Print and shaded views of the part. All mm, measured from the part's lowest x, y and z. A direction names the side the tool comes from. Coordinates: 2 decimals unless noted, no trailing zeros. Order: outer loops, then holes, each group sorted by start corner. A loop starts at its lowest first (then second) coordinate and runs counter-clockwise, first axis right, second up. Notation, with made-up numbers: (50.25, -31) -> (99.25, -31) arc R18 ccw to (99.25, -26) -> close; hole circle Ø4 at (44.5, -9.5). An arc over 180 degrees is marked (long way). Return JSON: item names as keys, results as strings. Group by question number.
1) Probe line 1 (X direction, y = 0.35, z = 4.75); line 2 (Z direction, x = 13, y = 0.8); line 3 (X direction, y = 2.9, z = 1.5). List the from-to ranges inside material, lowest first.
2) Cut at C-C (z = 1.5). Write the cut outline in (x, y), and give its area (3 significant figures).
3) Which spindle directions (+Z, -Z, +X, -X, +Y, -Y) get a long thin tool onto all of the face, cutting with end or side? Do the marked faces 4 and 5. Say none if no direction does.
4) Flat gauge pins, fed straight in: pin 1 (1 mm diameter, centred on y = 2, z = 5.5, fed in from +X); pin 2 (5 mm diameter, centred on x = 9.5, z = 6, fed in from +Y). Where does each tip first touch, or does it go through?
5) Cut at D-D (y = 0.4). Write the cut outline in (x, z), and give its area (3 significant figures).
6) Pull direction X, two halves, no side cores. Call the marked faces 1, 2 and 3: +X half, -X half, draft (parallel to the pull), parting line (faces both ways), or undercut.
7) Cut at B-B (x = 8). Write the cut outline in (y, z), and give its area (3 significant figures).
8) Cut at A-A (z = 4.75). Write the cut outline in (x, y), and give its area (3 significant figures).
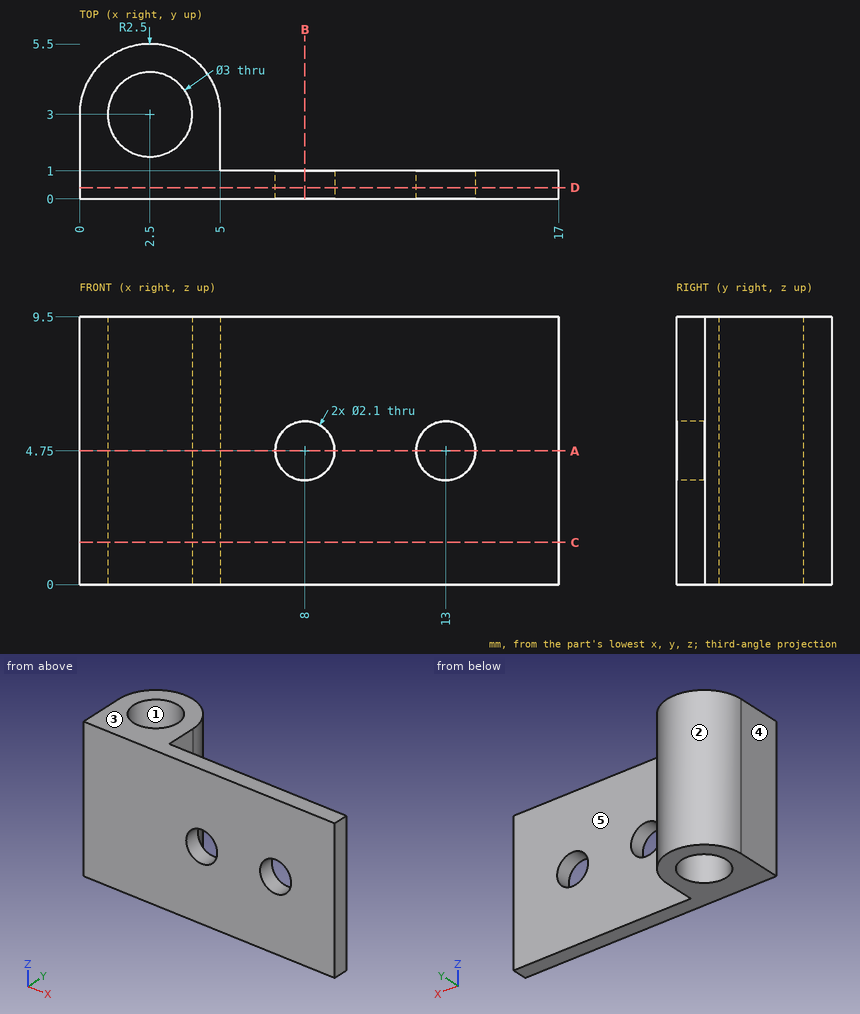
Answers below:
{
 "1": {"line 1": "x = 0 to 6.95, 9.05 to 11.95, 14.05 to 17", "line 2": "z = 0 to 3.7, 5.8 to 9.5", "line 3": "x = 0 to 1, 4 to 5"},
 "2": {"outline": "(0, 0) -> (17, 0) -> (17, 1) -> (5, 1) -> (5, 3) arc R2.5 ccw to (0, 3) -> close; hole circle Ø3 at (2.5, 3)", "area": "29.7 mm^2"},
 "3": {"face 4": "+Z, -Z, -X, +Y, -Y", "face 5": "+Z, -Z, +X, +Y"},
 "4": {"pin 1": "stops at x = 5", "pin 2": "stops at y = 1"},
 "5": {"outline": "(0, 0) -> (17, 0) -> (17, 9.5) -> (0, 9.5) -> close; hole circle Ø2.1 at (8, 4.75); hole circle Ø2.1 at (13, 4.75)", "area": "155 mm^2"},
 "6": {"face 1": "undercut", "face 2": "parting line", "face 3": "draft"},
 "7": {"outline": "(0, 0) -> (1, 0) -> (1, 3.7) -> (0, 3.7) -> close; (0, 5.8) -> (1, 5.8) -> (1, 9.5) -> (0, 9.5) -> close", "area": "7.40 mm^2"},
 "8": {"outline": "(0, 0) -> (6.95, 0) -> (6.95, 1) -> (5, 1) -> (5, 3) arc R2.5 ccw to (0, 3) -> close; (9.05, 0) -> (11.95, 0) -> (11.95, 1) -> (9.05, 1) -> close; (14.05, 0) -> (17, 0) -> (17, 1) -> (14.05, 1) -> close; hole circle Ø3 at (2.5, 3)", "area": "25.5 mm^2"}
}
